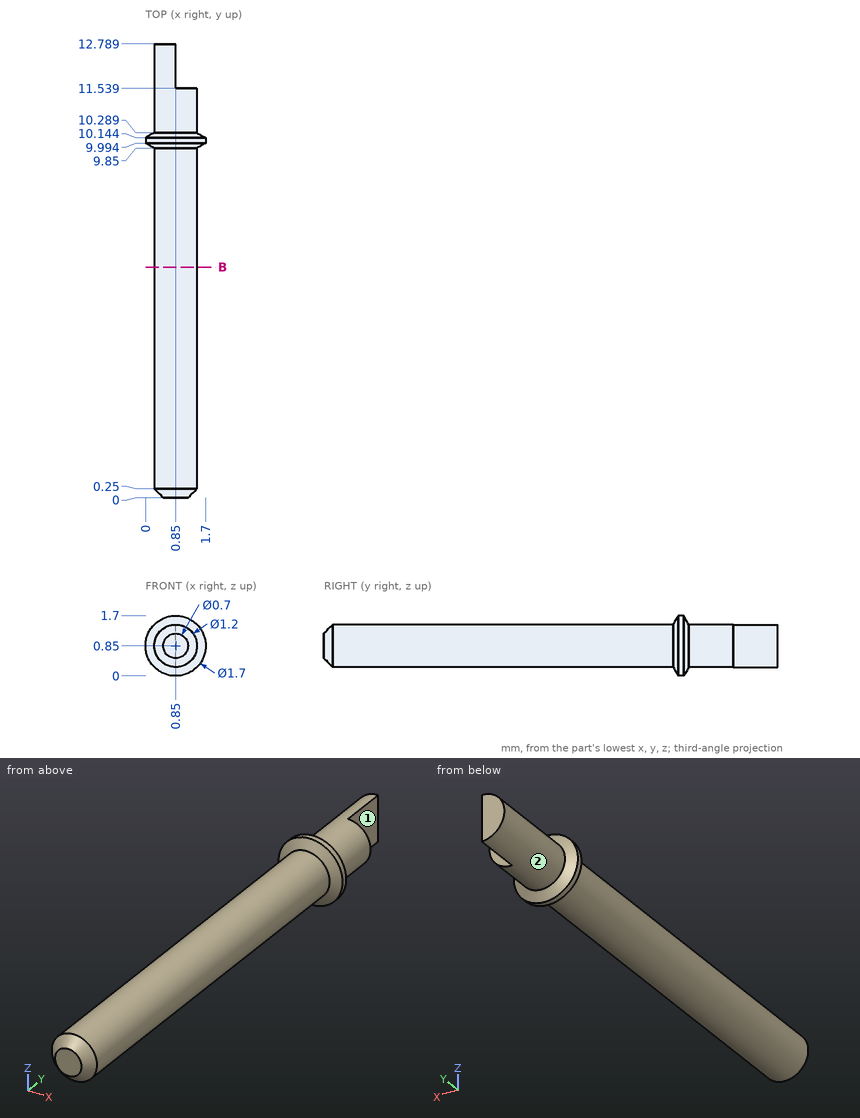
Study the drawing (mm; zero at the part's minimum x, y, z) and answer. Give positions to 0.01 mm unless a question says otherwise; leave off trailing zeros. Write each loop counter-clockwise with the first axis right and the second up, starting at its lowest first coordinate (ties: lowest second). Pieces come first, ordered by that corner, then holes.
Item 1: A flat-ended cylindrical pin translates along its axis: P1, Ø0.6, axis at y = 12, z = 1, coming from the +X side. Find the tip coordinate at first contact, or state that the pin passes through.
Item 2: Determine the mould class of the marked faces 1 and 2 for opening direction X: released by +X, released by -X, zero draft, split by the parting line, or undercut.
Item 3: Section B-B, the plane y = 6.5 is taken. Write down the section's boundary in (x, z), plus the area to 3 significant figures.
Item 4: Find the intervals of material crossed by line 1 along X through (y, z) = (3.5, 0.8); line 2 along X through (y, z) = (2.5, 1.3) (1 decimal); line 3 along Z through (x, y) = (1.2, 3.75), in increasing order.
Completed:
1. P1: stops at x = 0.85
2. face 1: released by +X
2. face 2: split by the parting line
3. outline: circle Ø1.2 at (0.85, 0.85)
3. area: 1.13 mm2
4. line 1: x = 0.25 to 1.45
4. line 2: x = 0.5 to 1.2
4. line 3: z = 0.36 to 1.34
